Part model, mm, in its own coordinate system. A direction names the side the tool comes from. Coordinates: 2 decimals unless noted, no trailing zeros. Write each loop counter-clockwise with the first axis right and the second up, starting at its lowest first coordinate (ties: lowest second). Pieces come first, ordered by that corner, then holes. Notation, with made-up numbers: (-37, 50) - (-30, 50) arc R27 ccw to (-30, 71) - close; hole circle Ø4 at (80.5, 34.5). An arc over 180 degrees is marked (long way). Use a Markdown table: item, result.
```python
from build123d import *

# Parameters (mm, degrees)
BOSS_EXTRUDE1_DEPTH   = 11.4
BOSS_EXTRUDE1_2_DEPTH = 11.4
BOSS_EXTRUDE1_3_DEPTH = 11.4
BOSS_EXTRUDE1_4_DEPTH = 11.4
BOSS_EXTRUDE1_5_DEPTH = 11.4
BOSS_EXTRUDE1_6_DEPTH = 11.4
BOSS_EXTRUDE2_START   = -20
SKETCH1_6_R           = 15.6
SKETCH1_6_R_2         = 10
BOSS_EXTRUDE2_DEPTH   = 20
SKETCH2_R             = 2.75
CUT_EXTRUDE1_DEPTH    = 30


with BuildPart() as part:
    # Sketch1 → Boss-Extrude1 (new body)
    with BuildSketch(Plane.XY):
        with BuildLine():
            ThreePointArc((-4.460468257, 14.948719776), (-0.063074903, 15.599872485), (4.339440194, 14.984300411))
            Line((4.339440194, 14.984300411), (4.339440194, 21.56778289))
            ThreePointArc((4.339440194, 21.56778289), (-0.061761858, 21.999913306), (-4.460468257, 21.543078307))
            Line((-4.460468257, 21.543078307), (-4.460468257, 14.948719776))
        make_face()
    extrude(amount=BOSS_EXTRUDE1_DEPTH)



with BuildPart() as body_2:
    # Sketch1 → Boss-Extrude1 2 (new body)
    with BuildSketch(Plane.XY):
        with BuildLine():
            Line((16.426618961, 14.634417977), (10.715736951, 11.337238711))
            ThreePointArc((10.715736951, 11.337238711), (13.478348416, 7.854560711), (15.146504911, 3.734084759))
            Line((15.146504911, 3.734084759), (20.847967983, 7.025825999))
            ThreePointArc((20.847967983, 7.025825999), (19.021602875, 11.053443991), (16.426618961, 14.634417977))
        make_face()
    extrude(amount=BOSS_EXTRUDE1_2_DEPTH)


with BuildPart() as body_3:
    # Sketch1 → Boss-Extrude1 3 (new body)
    with BuildSketch(Plane.XY):
        with BuildLine():
            Line((20.887087218, -6.90866033), (15.176205208, -3.611481064))
            ThreePointArc((15.176205208, -3.611481064), (13.54142332, -7.745311774), (10.807064717, -11.250215651))
            Line((10.807064717, -11.250215651), (16.508527789, -14.541956891))
            ThreePointArc((16.508527789, -14.541956891), (19.083364733, -10.946469315), (20.887087218, -6.90866033))
        make_face()
    extrude(amount=BOSS_EXTRUDE1_3_DEPTH)


with BuildPart() as body_4:
    # Sketch1 → Boss-Extrude1 4 (new body)
    with BuildSketch(Plane.XY):
        with BuildLine():
            Line((4.460468257, -21.543078307), (4.460468257, -14.948719776))
            ThreePointArc((4.460468257, -14.948719776), (0.063074903, -15.599872485), (-4.339440194, -14.984300411))
            Line((-4.339440194, -14.984300411), (-4.339440194, -21.56778289))
            ThreePointArc((-4.339440194, -21.56778289), (0.061761858, -21.999913306), (4.460468257, -21.543078307))
        make_face()
    extrude(amount=BOSS_EXTRUDE1_4_DEPTH)


with BuildPart() as body_5:
    # Sketch1 → Boss-Extrude1 5 (new body)
    with BuildSketch(Plane.XY):
        with BuildLine():
            ThreePointArc((-10.715736951, -11.337238711), (-13.478348416, -7.854560711), (-15.146504911, -3.734084759))
            Line((-15.146504911, -3.734084759), (-20.847967983, -7.025825999))
            ThreePointArc((-20.847967983, -7.025825999), (-19.021602875, -11.053443991), (-16.426618961, -14.634417977))
            Line((-16.426618961, -14.634417977), (-10.715736951, -11.337238711))
        make_face()
    extrude(amount=BOSS_EXTRUDE1_5_DEPTH)


with BuildPart() as body_6:
    # Sketch1 → Boss-Extrude1 6 (new body)
    with BuildSketch(Plane.XY):
        with BuildLine():
            ThreePointArc((-15.176205208, 3.611481064), (-13.54142332, 7.745311774), (-10.807064717, 11.250215651))
            Line((-10.807064717, 11.250215651), (-16.508527789, 14.541956891))
            ThreePointArc((-16.508527789, 14.541956891), (-19.083364733, 10.946469315), (-20.887087218, 6.90866033))
            Line((-20.887087218, 6.90866033), (-15.176205208, 3.611481064))
        make_face()
    extrude(amount=BOSS_EXTRUDE1_6_DEPTH)


with BuildPart() as part_1:
    add(part.part)

    add(body_2.part)  # Boss-Extrude2 merges body 2

    add(body_3.part)  # Boss-Extrude2 merges body 3

    add(body_4.part)  # Boss-Extrude2 merges body 4

    add(body_5.part)  # Boss-Extrude2 merges body 5

    add(body_6.part)  # Boss-Extrude2 merges body 6
    # Sketch1_6 → Boss-Extrude2 (add)
    # profile 1 of 14: a face of its own
    with BuildSketch(Plane.XY.offset(BOSS_EXTRUDE2_START)):
        with BuildLine():
            Line((4.339440194, 21.56778289), (4.339440194, 14.984300411))
            ThreePointArc((4.339440194, 14.984300411), (7.745311774, 13.54142332), (10.715736951, 11.337238711))
            Line((10.715736951, 11.337238711), (16.426618961, 14.634417977))
            ThreePointArc((16.426618961, 14.634417977), (10.946469315, 19.083364733), (4.339440194, 21.56778289))
        make_face()
    # profile 2 of 14: a face of its own
    with BuildSketch(Plane.XY.offset(BOSS_EXTRUDE2_START)):
        with BuildLine():
            ThreePointArc((-4.460468257, 14.948719776), (-0.063074903, 15.599872485), (4.339440194, 14.984300411))
            Line((4.339440194, 14.984300411), (4.339440194, 21.56778289))
            ThreePointArc((4.339440194, 21.56778289), (-0.061761858, 21.999913306), (-4.460468257, 21.543078307))
            Line((-4.460468257, 21.543078307), (-4.460468257, 14.948719776))
        make_face()
    # profile 3 of 14: a face of its own
    with BuildSketch(Plane.XY.offset(BOSS_EXTRUDE2_START)):
        with BuildLine():
            ThreePointArc((-10.807064717, 11.250215651), (-7.854560711, 13.478348416), (-4.460468257, 14.948719776))
            Line((-4.460468257, 14.948719776), (-4.460468257, 21.543078307))
            ThreePointArc((-4.460468257, 21.543078307), (-11.053443991, 19.021602875), (-16.508527789, 14.541956891))
            Line((-16.508527789, 14.541956891), (-10.807064717, 11.250215651))
        make_face()
    # profile 4 of 14: a face of its own
    with BuildSketch(Plane.XY.offset(BOSS_EXTRUDE2_START)):
        with BuildLine():
            ThreePointArc((-15.176205208, 3.611481064), (-13.54142332, 7.745311774), (-10.807064717, 11.250215651))
            Line((-10.807064717, 11.250215651), (-16.508527789, 14.541956891))
            ThreePointArc((-16.508527789, 14.541956891), (-19.083364733, 10.946469315), (-20.887087218, 6.90866033))
            Line((-20.887087218, 6.90866033), (-15.176205208, 3.611481064))
        make_face()
    # profile 5 of 14: a face of its own
    with BuildSketch(Plane.XY.offset(BOSS_EXTRUDE2_START)):
        with BuildLine():
            ThreePointArc((-15.146504911, -3.734084759), (-15.599872485, -0.063074903), (-15.176205208, 3.611481064))
            Line((-15.176205208, 3.611481064), (-20.887087218, 6.90866033))
            ThreePointArc((-20.887087218, 6.90866033), (-21.999913306, -0.061761858), (-20.847967983, -7.025825999))
            Line((-20.847967983, -7.025825999), (-15.146504911, -3.734084759))
        make_face()
    # profile 6 of 14: a face of its own
    with BuildSketch(Plane.XY.offset(BOSS_EXTRUDE2_START)):
        with BuildLine():
            ThreePointArc((-10.715736951, -11.337238711), (-13.478348416, -7.854560711), (-15.146504911, -3.734084759))
            Line((-15.146504911, -3.734084759), (-20.847967983, -7.025825999))
            ThreePointArc((-20.847967983, -7.025825999), (-19.021602875, -11.053443991), (-16.426618961, -14.634417977))
            Line((-16.426618961, -14.634417977), (-10.715736951, -11.337238711))
        make_face()
    # profile 7 of 14: a face of its own
    with BuildSketch(Plane.XY.offset(BOSS_EXTRUDE2_START)):
        with BuildLine():
            ThreePointArc((-4.339440194, -14.984300411), (-7.745311774, -13.54142332), (-10.715736951, -11.337238711))
            Line((-10.715736951, -11.337238711), (-16.426618961, -14.634417977))
            ThreePointArc((-16.426618961, -14.634417977), (-10.946469315, -19.083364733), (-4.339440194, -21.56778289))
            Line((-4.339440194, -21.56778289), (-4.339440194, -14.984300411))
        make_face()
    # profile 8 of 14: a face of its own
    with BuildSketch(Plane.XY.offset(BOSS_EXTRUDE2_START)):
        with BuildLine():
            Line((4.460468257, -21.543078307), (4.460468257, -14.948719776))
            ThreePointArc((4.460468257, -14.948719776), (0.063074903, -15.599872485), (-4.339440194, -14.984300411))
            Line((-4.339440194, -14.984300411), (-4.339440194, -21.56778289))
            ThreePointArc((-4.339440194, -21.56778289), (0.061761858, -21.999913306), (4.460468257, -21.543078307))
        make_face()
    # profile 9 of 14: a face of its own
    with BuildSketch(Plane.XY.offset(BOSS_EXTRUDE2_START)):
        with BuildLine():
            Line((16.508527789, -14.541956891), (10.807064717, -11.250215651))
            ThreePointArc((10.807064717, -11.250215651), (7.854560711, -13.478348416), (4.460468257, -14.948719776))
            Line((4.460468257, -14.948719776), (4.460468257, -21.543078307))
            ThreePointArc((4.460468257, -21.543078307), (11.053443991, -19.021602875), (16.508527789, -14.541956891))
        make_face()
    # profile 10 of 14: a face of its own
    with BuildSketch(Plane.XY.offset(BOSS_EXTRUDE2_START)):
        with BuildLine():
            Line((20.887087218, -6.90866033), (15.176205208, -3.611481064))
            ThreePointArc((15.176205208, -3.611481064), (13.54142332, -7.745311774), (10.807064717, -11.250215651))
            Line((10.807064717, -11.250215651), (16.508527789, -14.541956891))
            ThreePointArc((16.508527789, -14.541956891), (19.083364733, -10.946469315), (20.887087218, -6.90866033))
        make_face()
    # profile 11 of 14: a face of its own
    with BuildSketch(Plane.XY.offset(BOSS_EXTRUDE2_START)):
        with BuildLine():
            Line((20.847967983, 7.025825999), (15.146504911, 3.734084759))
            ThreePointArc((15.146504911, 3.734084759), (15.486211231, 1.880760936), (15.6, 0))
            ThreePointArc((15.6, 0), (15.493689058, -1.818130737), (15.176205208, -3.611481064))
            Line((15.176205208, -3.611481064), (20.887087218, -6.90866033))
            ThreePointArc((20.887087218, -6.90866033), (21.719989857, -3.498862759), (22, 0))
            ThreePointArc((22, 0), (21.710081709, 3.559824741), (20.847967983, 7.025825999))
        make_face()
    # profile 12 of 14: a face of its own
    with BuildSketch(Plane.XY.offset(BOSS_EXTRUDE2_START)):
        with BuildLine():
            Line((16.426618961, 14.634417977), (10.715736951, 11.337238711))
            ThreePointArc((10.715736951, 11.337238711), (13.478348416, 7.854560711), (15.146504911, 3.734084759))
            Line((15.146504911, 3.734084759), (20.847967983, 7.025825999))
            ThreePointArc((20.847967983, 7.025825999), (19.021602875, 11.053443991), (16.426618961, 14.634417977))
        make_face()
    # profile 13 of 14: a face of its own
    with BuildSketch(Plane.XY.offset(BOSS_EXTRUDE2_START)):
        Circle(SKETCH1_6_R)
        Circle(SKETCH1_6_R_2, mode=Mode.SUBTRACT)
    # profile 14 of 14: a face of its own
    with BuildSketch(Plane.XY.offset(BOSS_EXTRUDE2_START)):
        Circle(SKETCH1_6_R_2)
        with BuildLine():
            ThreePointArc((-2.828427125, 3.5), (0, -4.5), (2.828427125, 3.5))
            Line((2.828427125, 3.5), (-2.828427125, 3.5))
        make_face(mode=Mode.SUBTRACT)
    extrude(amount=BOSS_EXTRUDE2_DEPTH)

    # Sketch2 → Cut-Extrude1 (cut)
    with BuildSketch(Plane(origin=(0, 0, 0), x_dir=(1, 0, 0), z_dir=(0, 1, 0))):
        with Locations(Location((0, 12.5, 0), (0, 0, 90))):
            Circle(SKETCH2_R)
    extrude(amount=CUT_EXTRUDE1_DEPTH, mode=Mode.SUBTRACT)


solid = part_1.part
```
Item 1: Band-saw the part on B-B, the plane x = 0. Give the cut face in (y, z), then the cut area to 3 significant figures.
From the geometry:
| item | result |
|---|---|
| outline | (-22, -20) - (-4.5, -20) - (-4.5, 0) - (-15.6, 0) - (-15.6, 11.4) - (-22, 11.4) - close; (3.5, -20) - (22, -20) - (22, -15.25) - (3.5, -15.25) - close; (3.5, -9.75) - (22, -9.75) - (22, 11.4) - (15.6, 11.4) - (15.6, 0) - (3.5, 0) - close |
| area | 764 mm^2 |
Item 2: Band-saw the part on D-D, the plane z = -1.5. Give the cut face in (x, y).
From the geometry:
| item | result |
|---|---|
| outline | circle Ø44 at (0, 0); hole (-2.83, 3.5) arc R4.5 ccw (long way) to (2.83, 3.5) - close |
Item 3: Band-saw the part on A-A, the plane z = 6. Give the cut face in (x, y), then the cut area to 3 significant figures.
From the geometry:
| item | result |
|---|---|
| outline | (-20.89, 6.91) - (-15.18, 3.61) arc R15.6 cw to (-10.81, 11.25) - (-16.51, 14.54) arc R22 ccw to start; (-20.85, -7.03) arc R22 ccw to (-16.43, -14.63) - (-10.72, -11.34) arc R15.6 cw to (-15.15, -3.73) - close; (-4.46, 14.95) arc R15.6 cw to (4.34, 14.98) - (4.34, 21.57) arc R22 ccw to (-4.46, 21.54) - close; (-4.34, -21.57) arc R22 ccw to (4.46, -21.54) - (4.46, -14.95) arc R15.6 cw to (-4.34, -14.98) - close; (10.72, 11.34) arc R15.6 cw to (15.15, 3.73) - (20.85, 7.03) arc R22 ccw to (16.43, 14.63) - close; (10.81, -11.25) - (16.51, -14.54) arc R22 ccw to (20.89, -6.91) - (15.18, -3.61) arc R15.6 cw to start |
| area | 341 mm^2 |
Item 4: Drill centre lines: probe 1 along Y at (x, z) = (0, -4); probe 2 along Z at (x, y) = (13, 6.5); probe 3 along Z at (x, y) = (-2, 20.5). Where is each one in solid material? Low to high.
From the geometry:
| item | result |
|---|---|
| probe 1 | -22 to -4.5, 3.5 to 22 |
| probe 2 | -20 to 0 |
| probe 3 | -20 to -14.39, -10.61 to 11.4 |
Item 5: Drop flat-ended pins along their axis: P1, Ø3, axis at x = -9, y = -13.5, coming from the +Z side; P2, Ø8, axis at x = -14, y = 16, coming from the +Z side; P3, Ø5.5, axis at y = 18.5, z = 3, coming from the +X side; P4, Ø3.5, axis at y = -17, z = 7, coming from the -X side. Give the stop position or say it passes through.
From the geometry:
| item | result |
|---|---|
| P1 | z = 0 |
| P2 | z = 11.4 |
| P3 | x = 4.34 |
| P4 | x = -4.34 |
Item 6: Which spindle directions (+Z, -Z, +X, -X, +Y, -Y) get a long thin tool onto all of the face, cutting with end or side? Do faces 1 (the face through (-18.1, 5.3, 5.6)), 2 (the face through (4.46, -18, 6)), 3 (the face through (-13.447, -7.908, 5.62)). Say none if no direction does.
From the geometry:
| item | result |
|---|---|
| face 1 | +Z, -X |
| face 2 | +Z, +X, +Y, -Y |
| face 3 | +Z |
Item 7: Two-plate mould, pull along X, no slides. Class faces 4 (the face through (13.447, 7.908, 5.62)), 5 (the face through (16, -9, 11.4)), 6 (the face through (17.96, 5.36, 5.62)): pulls with the +X half, pulls with the -X half, needs draft (parallel to the pull), parting line crosses it, or undercut.
From the geometry:
| item | result |
|---|---|
| face 4 | undercut |
| face 5 | needs draft |
| face 6 | pulls with the +X half |
Item 8: Band-saw the part on C-C, the plane y = -1. Give the cut face in (x, z), then the cut area to 3 significant figures.
From the geometry:
| item | result |
|---|---|
| outline | (-21.98, -20) - (-4.39, -20) - (-4.39, 0) - (-21.98, 0) - close; (4.39, -20) - (21.98, -20) - (21.98, 0) - (4.39, 0) - close |
| area | 704 mm^2 |
